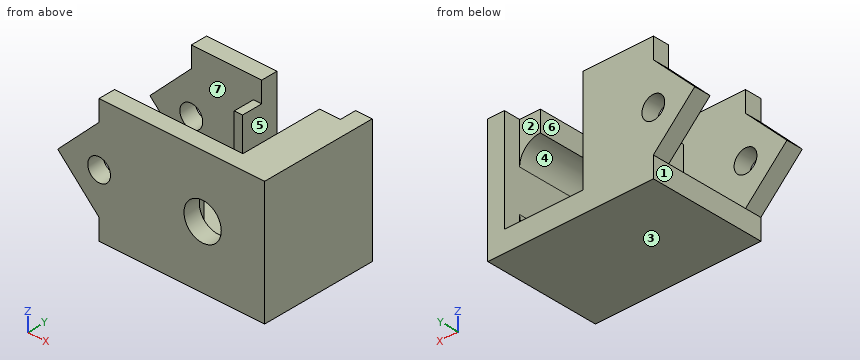
from build123d import *

# Parameters (mm, degrees)
SKETCH058_W     = 50
SKETCH058_H     = 30
PAD015_DEPTH    = 28
SKETCH059_R     = 4.5
HOLE009_DEPTH   = 4
HOLE009_TIPS_R  = 4.5
SKETCH060_W     = 20
SKETCH060_H     = 20
POCKET021_DEPTH = 46
POCKET022_DEPTH = 28.001
SKETCH062_R     = 2.75
HOLE010_DEPTH   = 28.001
SKETCH063_W     = 42
SKETCH063_H     = 20
POCKET023_DEPTH = 25
SKETCH064_W     = 2
SKETCH064_H     = 20
PAD016_DEPTH    = 5
PAD017_DEPTH    = 24
SKETCH066_W     = 5
SKETCH066_H     = 5
PAD018_DEPTH    = 20
SKETCH067_W     = 19
SKETCH067_H     = 25
POCKET024_DEPTH = 4
SKETCH068_W     = 2
SKETCH068_H     = 20
PAD019_DEPTH    = 5


with BuildPart() as part:
    # Sketch058 → Pad015 (new body)
    with BuildSketch(Plane.XZ.offset(-144)):
        with Locations((150, 200)):
            Rectangle(SKETCH058_W, SKETCH058_H)
    extrude(amount=PAD015_DEPTH)

    # Sketch059 (on Face6 of Pad015) → Hole009 (cut)
    with BuildSketch(Plane.XZ.offset(-116)):
        with Locations((160, 200)):
            Circle(SKETCH059_R)
    extrude(amount=-HOLE009_DEPTH, mode=Mode.SUBTRACT)

    # Hole009 tips → Hole009 tip 1 section 0
    with BuildSketch(Plane.XZ.offset(-120), mode=Mode.PRIVATE) as hole009_tip_1_s0:
        with Locations((160, 200)):
            Circle(HOLE009_TIPS_R)
    loft([hole009_tip_1_s0.sketch, Vertex(160, 122.703873, 200)], mode=Mode.SUBTRACT)

    # Sketch060 (on Face2 of Hole009) → Pocket021 (cut)
    with BuildSketch(Plane(origin=(125, 0, 0), x_dir=(0, 0, -1), z_dir=(-1, 0, 0))):
        with Locations((-200, -130)):
            Rectangle(SKETCH060_W, SKETCH060_H)
    extrude(amount=-POCKET021_DEPTH, mode=Mode.SUBTRACT)

    # Sketch061 (on Face5 of Pocket021) → Pocket022 (cut, through all)
    with BuildSketch(Plane.XZ.offset(-116)):
        Polygon((125, 200), (135, 190), (135, 185), (125, 185), (125, 215), (135, 215), (135, 210), align=None)
    extrude(amount=-POCKET022_DEPTH, mode=Mode.SUBTRACT)

    # Sketch062 (on Face4 of Pocket022) → Hole010 (cut, through all)
    with BuildSketch(Plane.XZ.offset(-116)):
        with Locations((135, 200)):
            Circle(SKETCH062_R)
    extrude(amount=-HOLE010_DEPTH, mode=Mode.SUBTRACT)

    # Sketch063 (on Face7 of Hole010) → Pocket023 (cut)
    with BuildSketch(Plane(origin=(0, 0, 215), x_dir=(-1, 0, 0), z_dir=(0, 0, 1))):
        with Locations((-150, -130)):
            Rectangle(SKETCH063_W, SKETCH063_H)
    extrude(amount=-POCKET023_DEPTH, mode=Mode.SUBTRACT)

    # Sketch064 (on Face23 of Pocket023) → Pad016 (join)
    with BuildSketch(Plane(origin=(0, 120, 0), x_dir=(1, 0, 0), z_dir=(0, 1, 0))):
        with Locations((151, -200)):
            Rectangle(SKETCH064_W, SKETCH064_H)
    extrude(amount=PAD016_DEPTH)

    # Sketch065 (on Face2 of Pocket023) → Pad017 (join)
    with BuildSketch(Plane(origin=(0, 144, 0), x_dir=(1, 0, 0), z_dir=(0, 1, 0))):
        with BuildLine():
            Line((166, -190), (171, -190))
            Line((171, -190), (171, -195))
            ThreePointArc((171, -195), (169.535534, -191.464466), (166, -190))
        make_face()
        with BuildLine():
            Line((166, -210), (171, -210))
            Line((171, -210), (171, -205))
            ThreePointArc((166, -210), (169.535534, -208.535534), (171, -205))
        make_face()
    extrude(amount=-PAD017_DEPTH)

    # Sketch066 (on Face21 of Pad017) → Pad018 (join)
    with BuildSketch(Plane.XZ.offset(-140)):
        with Locations((168.5, 212.5)):
            Rectangle(SKETCH066_W, SKETCH066_H)
    extrude(amount=PAD018_DEPTH)

    # Sketch067 (on Face2 of Pad018) → Pocket024 (cut)
    with BuildSketch(Plane(origin=(0, 144, 0), x_dir=(1, 0, 0), z_dir=(0, 1, 0))):
        with Locations((161.5, -202.5)):
            Rectangle(SKETCH067_W, SKETCH067_H)
    extrude(amount=-POCKET024_DEPTH, mode=Mode.SUBTRACT)

    # Sketch068 (on Face26 of Pocket024) → Pad019 (join)
    with BuildSketch(Plane.XZ.offset(-140)):
        with Locations((151, 200)):
            Rectangle(SKETCH068_W, SKETCH068_H)
    extrude(amount=PAD019_DEPTH)


solid = part.part
The model under review builds one solid part; all positions refer to its coordinate system, in mm. Face numbers are marked on the shaded views. A direction names the side the tool comes from. Give positions to 0.01 mm unless a question says otherwise; leave off trailing zeros. Write each loop counter-clockwise with the first axis right and the second up, starting at its lowest first coordinate (ties: lowest second). Pieces come first, ordered by that corner, then holes.
1. Add section B-B, the plane x = 158. Write out the cut boundary in (y, z), plus the area to 3 significant figures.
2. Add section D-D, the plane z = 196.25. Write out the cut boundary in (x, y).
3. Wall thickness on L1, parallel to Z at x = 160, y = 117.25; L2, parallel to Y at x = 136, z = 209.75; L3, parallel to X at y = 125.75, z = 198.25: over which ranges is each line inside the solid? List them lowest first.
4. Add section A-A, the plane y = 123.5. Write out the cut boundary in (x, z).
5. For P1, Ø5.5, axis at y = 124, z = 187.5, coming from the -X side; P2, Ø4, axis at y = 127.5, z = 212.5, coming from the -X side; P3, Ø5.5, axis at y = 136.5, z = 198.5, coming from the -X side, all flat-tipped, find the tip position at first contact; note any pin that passes through.
6. Draft analysis for pull direction X (two halves, no side actions). For the marked faces 1, 2 and 3, state which applies: +X half, -X half, draft (parallel to the pull), parting line (faces both ways), or undercut.
7. Add section C-C, the plane z = 201.25. Write out the cut boundary in (x, y).
8. Tool access review of the marked faces 4, 5, 6 and 7: name each direction out of +Z, -Z, +X, -X, +Y, -Y from which nothing blocks a thin tool from reaching the whole face with its end or side.
Worked answers:
1. outline: (116, 185) - (144, 185) - (144, 190) - (120, 190) - (120, 195.97) - (116, 195.97) - close; (116, 204.03) - (120, 204.03) - (120, 215) - (116, 215) - close
1. area: 208 mm2
2. outline: (128.75, 116) - (157.51, 116) - (157.51, 120) - (152, 120) - (152, 125) - (150, 125) - (150, 120) - (128.75, 120) - close; (128.75, 140) - (150, 140) - (150, 135) - (152, 135) - (152, 144) - (128.75, 144) - close; (162.49, 116) - (175, 116) - (175, 144) - (171, 144) - (171, 120) - (162.49, 120) - close
3. L1: z = 185 to 195.5, 204.5 to 215
3. L2: y = 116 to 120, 140 to 144
3. L3: x = 171 to 175
4. outline: (135, 185) - (175, 185) - (175, 215) - (166, 215) - (166, 210) arc R5 cw to (171, 205) - (171, 195) arc R5 cw to (166, 190) - (152, 190) - (152, 210) - (150, 210) - (150, 190) - (135, 190) - close
5. P1: stops at x = 135
5. P2: stops at x = 166
5. P3: stops at x = 150
6. face 1: -X half
6. face 2: undercut
6. face 3: draft
7. outline: (126.25, 116) - (132.55, 116) - (132.55, 120) - (126.25, 120) - close; (126.25, 140) - (132.55, 140) - (132.55, 144) - (126.25, 144) - close; (137.45, 116) - (155.68, 116) - (155.68, 120) - (152, 120) - (152, 125) - (150, 125) - (150, 120) - (137.45, 120) - close; (137.45, 140) - (150, 140) - (150, 135) - (152, 135) - (152, 144) - (137.45, 144) - close; (164.32, 116) - (175, 116) - (175, 144) - (171, 144) - (171, 120) - (164.32, 120) - close
8. face 4: +Y
8. face 5: +Z, +Y
8. face 6: +Z, -X, +Y
8. face 7: +Z, -X
